The listing builds one solid part. Answer for the finished solid, in the listing's coordinates (mm). A direction names the side the tool comes from. Round coordinates to 2 decimals unless told otherwise and drop trailing zeros. Write each loop counter-clockwise with the first axis right and the second up, starting at its lowest first coordinate (ties: lowest second). Pieces come first, ordered by that corner, then holes.
Item 1: Each of these flat-tipped pins is pushed along its axis until it touches: pin 1 (1 mm diameter, centred on x = -4, y = 3, fed in from -Z); pin 2 (2 mm diameter, centred on y = 1.5, z = 1.5, fed in from -X). Where does it stop, or does it pass through?
Item 2: Find section A-A on x = 0. Give the vertices of the cut face in (y, z).
Item 3: Find section D-D on z = 8. Give the vertices of the cut face in (x, y).
Item 4: Find section C-C on y = 0.6. Give the vertices of the cut face in (x, z), then the cut area to 3 significant figures.
Item 5: Find section B-B on z = 1.5. Give the vertices of the cut face in (x, y), then the cut area to 3 significant figures.
Item 6: Find the intervals of material crossed by probe 1 along X at (y, z) = (3.6, 0); probe 2 along Z at (x, y) = (0.25, 4.25); probe 3 along Z at (x, y) = (14, 0.7), in increasing order.
Item 7: For a pull along Z with two mould halves and no side action, classify faces 1 (the face through (-10, 2, 10)), 2 (the face through (-4.88, 2.46, -1.08)), 3 (the face through (-12, 3, 20)) as +Z half, -Z half, draft (parallel to the pull), parting line (faces both ways), or undercut.
Item 8: A tool of negligible diameter and unlimited length cuts with its end or side. For faces 4 (the face through (-14.666, 2, 22)), 5 (the face through (10, 2, 10)), from which of +Z, -Z, +X, -X, +Y, -Y can it reach the whole face along a straight path? Write none if from no direction.
```python
from build123d import *

# Parameters (mm, degrees)
SKETCH2_R           = 5
BOSS_EXTRUDE1_DEPTH = 5
SKETCH3_W           = 30
SKETCH3_H           = 5
BOSS_EXTRUDE2_DEPTH = 5


with BuildPart() as part:
    # Sketch2 → Boss-Extrude1 (new body)
    with BuildSketch(Plane(origin=(0, 0, 0), x_dir=(1, 0, 0), z_dir=(0, 1, 0))):
        with BuildLine():
            Line((-10, 0), (-10, -20))
            Line((-10, -20), (10, -20))
            Line((10, -20), (10, 0))
            ThreePointArc((10, 0), (0, 10), (-10, 0))
        make_face()
        with Locations(Location((0, 0, 0), (0, 0, 270))):
            Circle(SKETCH2_R, mode=Mode.SUBTRACT)
    extrude(amount=BOSS_EXTRUDE1_DEPTH)

    # Sketch3 → Boss-Extrude2 (add)
    with BuildSketch(Plane.XY.offset(20)):
        with Locations((0.334158143, 2.5)):
            Rectangle(SKETCH3_W, SKETCH3_H)
    extrude(amount=BOSS_EXTRUDE2_DEPTH)


solid = part.part
```
Check values:
1. pin 1: stops at z = -9.37
1. pin 2: stops at x = -10
2. outline: (0, -10) - (5, -10) - (5, -5) - (0, -5) - close; (0, 5) - (5, 5) - (5, 25) - (0, 25) - close
3. outline: (-10, 0) - (10, 0) - (10, 5) - (-10, 5) - close
4. outline: (-14.67, 20) - (-10, 20) - (-10, 0) arc R10 ccw to (10, 0) - (10, 20) - (15.33, 20) - (15.33, 25) - (-14.67, 25) - close; hole circle Ø10 at (0, 0)
4. area: 629 mm2
5. outline: (-10, 0) - (-4.77, 0) - (-4.77, 5) - (-10, 5) - close; (4.77, 0) - (10, 0) - (10, 5) - (4.77, 5) - close
5. area: 52.3 mm2
6. probe 1: x = -10 to -5, 5 to 10
6. probe 2: z = -10 to -4.99, 4.99 to 25
6. probe 3: z = 20 to 25
7. face 1: draft
7. face 2: undercut
7. face 3: -Z half
8. face 4: +Z, -Z, -X, +Y, -Y
8. face 5: -Z, +X, +Y, -Y
